Part model, mm, in its own coordinate system. A direction names the side the tool comes from. Coordinates: 2 decimals unless noted, no trailing zeros. Write each loop counter-clockwise with the first axis right and the second up, starting at its lowest first coordinate (ties: lowest second). Pieces come first, ordered by that corner, then holes. Notation, with made-up numbers: (9, -12) - (44, -12) arc R20 cw to (44, 12) - close; hole circle Ø3 at (39, 31.5). An arc over 180 degrees is marked (long way). Write each question's results on one line, items separated by ' | '.
from build123d import *

# Parameters (mm, degrees)
SKETCH1_W                      = 25.4
SKETCH1_H                      = 25.4
EXTRUDE1_DEPTH                 = 6.096
SKETCH2_R                      = 11.938
EXTRUDE2_DEPTH                 = 58.42
SKETCH3_R                      = 3.175
EXTRUDE3_DEPTH                 = 18.796
F_4_40_TAPPED_HOLE3_D          = 2.2606
F_4_40_TAPPED_HOLE3_DEPTH      = 3.048
F_4_40_TAPPED_HOLE3_TIP        = 0.679152758
F_4_40_TAPPED_HOLE4_AT_2_COUNT = 2
F_4_40_TAPPED_HOLE4_AT_2_PITCH = 12.7
CIRPATTERN1_COUNT              = 4


with BuildPart() as part:
    # Sketch1 → Extrude1 (new body)
    with BuildSketch(Plane(origin=(0, 0, 0), x_dir=(1, 0, 0), z_dir=(0, 1, 0))):
        Rectangle(SKETCH1_W, SKETCH1_H)
    extrude(amount=EXTRUDE1_DEPTH)

    # Sketch2 → Extrude2 (add)
    with BuildSketch(Plane(origin=(0, 6.096, 0), x_dir=(1, 0, 0), z_dir=(0, 1, 0))):
        with Locations(Location((0, 0, 0), (0, 0, 270))):  # turned: the seam where the file's is
            Circle(SKETCH2_R)
    extrude(amount=EXTRUDE2_DEPTH)

    # Sketch3 → Extrude3 (add)
    with BuildSketch(Plane.XZ):
        with Locations(Location((0, 0, 0), (0, 0, 90))):  # turned: the seam where the file's is
            Circle(SKETCH3_R)
    extrude(amount=EXTRUDE3_DEPTH)

    # #4-40 Tapped Hole3
    with Locations(Plane(origin=(6.35, 0, -6.35), x_dir=(0, 0, -1), z_dir=(0, -1, 0))):
        with Locations((0, 0), (-12.7, 0), (-12.7, -12.7), (0, -12.7)):
            Hole(F_4_40_TAPPED_HOLE3_D / 2, depth=F_4_40_TAPPED_HOLE3_DEPTH)
            with Locations((0, 0, -(F_4_40_TAPPED_HOLE3_DEPTH + F_4_40_TAPPED_HOLE3_TIP / 2))):  # 118° drill point
                Cone(0, F_4_40_TAPPED_HOLE3_D / 2, F_4_40_TAPPED_HOLE3_TIP, mode=Mode.SUBTRACT)

    # Sketch12 → #4-40 Tapped Hole4 (revolve, cut)
    with BuildSketch(Plane(origin=(-12.7, 3.048, -6.35), x_dir=(0, 0, 1), z_dir=(0, 1, 0))):
        Polygon((0, 0), (0, 4.870152758), (1.1303, 4.191), (1.1303, 0), align=None)
    f_4_40_tapped_hole4 = revolve(axis=Axis((-19.05, 3.048, -6.35), (1, 0, 0)), mode=Mode.SUBTRACT)

    # #4-40 Tapped Hole4 at 2: #4-40 Tapped Hole4 ×2
    with Locations(*[(0, 0, i * F_4_40_TAPPED_HOLE4_AT_2_PITCH) for i in range(1, F_4_40_TAPPED_HOLE4_AT_2_COUNT)]):
        add(f_4_40_tapped_hole4, mode=Mode.SUBTRACT)

    # CirPattern1: #4-40 Tapped Hole4 ×4 about axis
    cirpattern1_axis = Axis((0, -18.796, 0), (0, 1, 0))
    for i in range(1, CIRPATTERN1_COUNT):
        add(f_4_40_tapped_hole4.rotate(cirpattern1_axis, i * 360 / CIRPATTERN1_COUNT), mode=Mode.SUBTRACT)

    # CirPattern1 copy 1 sketch → CirPattern1 copy 1 (revolve, cut)
    with BuildSketch(Plane(origin=(6.35, 3.048, 12.7), x_dir=(1, 0, 0), z_dir=(0, 1, 0))):
        Polygon((0, 0), (0, 4.870152758), (1.1303, 4.191), (1.1303, 0), align=None)
    revolve(axis=Axis((6.35, 3.048, 19.05), (0, 0, -1)), mode=Mode.SUBTRACT)

    # CirPattern1 copy 2 sketch → CirPattern1 copy 2 (revolve, cut)
    with BuildSketch(Plane(origin=(12.7, 3.048, -6.35), x_dir=(0, 0, -1), z_dir=(0, 1, 0))):
        Polygon((0, 0), (0, 4.870152758), (1.1303, 4.191), (1.1303, 0), align=None)
    revolve(axis=Axis((19.05, 3.048, -6.35), (-1, 0, 0)), mode=Mode.SUBTRACT)

    # CirPattern1 copy 3 sketch → CirPattern1 copy 3 (revolve, cut)
    with BuildSketch(Plane(origin=(-6.35, 3.048, -12.7), x_dir=(-1, 0, 0), z_dir=(0, 1, 0))):
        Polygon((0, 0), (0, 4.870152758), (1.1303, 4.191), (1.1303, 0), align=None)
    revolve(axis=Axis((-6.35, 3.048, -19.05), (0, 0, 1)), mode=Mode.SUBTRACT)

    # Sketch13 → Cut-Revolve1 (revolve, cut)
    with BuildSketch(Plane.XY, mode=Mode.PRIVATE) as cut_revolve1_sk:
        Polygon((-11.938, 25.542875), (-11.541125, 25.146), (-11.938, 24.749125), align=None)
    revolve(cut_revolve1_sk.sketch.rotate(Axis((0, 64.516, 0), (0, -1, 0)), 270), axis=Axis((0, 64.516, 0), (0, -1, 0)), mode=Mode.SUBTRACT)  # turned: the seam where the file's is


solid = part.part
(1) Saw through at D-D on y = 55. Write the cut outline in (x, z), then the cut area to 3 significant figures.
Return value:
outline: circle Ø23.88 at (0, 0) | area: 448 mm^2
(2) Saw through at A-A on y = -10. Write the cut outline in (x, z) (3 decimals), then the cut area to 3 significant figures.
Return value:
outline: circle Ø6.35 at (0, 0) | area: 31.7 mm^2
(3) Wall check: line 1 (Z direction, x = -6.35, y = 1.5); line 2 (Y direction, x = 10.05, z = 6.35). Give the ranges that are in metal, low to high. Write a range as from..to.
Return value:
line 1: z = -12.7..-7.48, -5.22..5.22, 7.48..12.7 | line 2: y = 0..1.92, 4.18..24.8, 25.49..64.52
(4) Flat gauge pins, fed straight in: P1, Ø3, axis at x = 8.5, y = 11.5, coming from the -Z side; P2, Ø2.5, axis at y = 3.048, z = -6.35, coming from the +X side; P3, Ø5, axis at y = 30.5, z = -4, coming from the +X side; P4, Ø12, axis at x = -5, y = 26, coming from the -Z side. Where does each tip first touch, or does it go through?
Return value:
P1: stops at z = -9.67 | P2: stops at x = 12.7 | P3: stops at x = 11.84 | P4: stops at z = -11.94
(5) Saw through at B-B on x = 0. Write the cut outline in (y, z) (3 decimals).
Return value:
outline: (-18.796, -3.175) - (0, -3.175) - (0, -12.7) - (6.096, -12.7) - (6.096, -11.938) - (24.749, -11.938) - (25.146, -11.541) - (25.543, -11.938) - (64.516, -11.938) - (64.516, 11.938) - (25.543, 11.938) - (25.146, 11.541) - (24.749, 11.938) - (6.096, 11.938) - (6.096, 12.7) - (0, 12.7) - (0, 3.175) - (-18.796, 3.175) - close
(6) 3-axis set-ups, long thin cutter, end or side, ignore diameter. For faces 5 (the flat face through (-9.5, 6.096, 7.5)), 6 (the cylindrical face through (-5.306, 3.481, 10.634)), 7 (the cylindrical face through (-5.22, 3, -10.63)), 8 (the cylindrical face through (-10.63, 3, 5.22)): which of +Z, -Z, +X, -X, +Y, -Y reach the whole face in a straight line?
Return value:
face 5: +Y | face 6: +Z | face 7: -Z | face 8: -X
(7) Saw through at C-C on x = 10. Count the separate pieces of the cut face and the enclosed holes in it, then the cut area to 3 significant figures.
Return value:
separate pieces: 1 | enclosed holes: 2 | area: 908 mm^2
(8) Two-plate mould, pull along X, no slides. Class faces 1 (the cylindrical face through (-10.63, 4.15, -6.6)), 2 (the conical face through (-7.95, 3.04, 6.15)), 3 (the conical face through (7.95, 3.04, -6.15)), 4 (the conical face through (6.15, 3.04, 7.95)): released by +X, released by -X, zero draft, split by the parting line, or undercut.
Return value:
face 1: zero draft | face 2: released by -X | face 3: released by +X | face 4: undercut
